```python
from build123d import *

# Parameters (mm, degrees)
F0_W     = 70
F0_H     = 100
F1_DEPTH = 10
F3_DEPTH = 70
F4_R     = 5
F6_D     = 11
F9_DEPTH = 17.2


with BuildPart() as f1:
    # F0 (on Front) → F1 (new body)
    with BuildSketch(Plane.XZ):
        with Locations((-0.1439042389, 3.7611486804)):
            Rectangle(F0_W, F0_H)
    extrude(amount=F1_DEPTH)

    # F2 (on face) → F3 (join)
    with BuildSketch(Plane.YZ.offset(34.8560957611)):
        with BuildLine():
            Line((-10, -46.2388513196), (-10, 53.7611486804))
            ThreePointArc((-10, 53.7611486804), (-21.8296936781, 3.7611486804), (-10, -46.2388513196))
        make_face()
    extrude(amount=-F3_DEPTH)

    # F4
    f4_edges = [f1.edges().sort_by_distance(p)[0] for p in [
        (34.856096, -5, 53.761149),
        (-35.143904, -5, 53.761149),
        (34.856096, -5, -46.238851),
        (-35.143904, -5, -46.238851),
    ]]
    fillet(f4_edges, radius=F4_R)

    # F6 (through all)
    with Locations(Plane(origin=(0, 0, 0), x_dir=(1, 0, 0), z_dir=(0, 1, 0))):
        with Locations((0, -33.7616663978), (0, -21.2616663978), (0, 13.7393690371), (0, 26.2393690371)):
            Hole(F6_D / 2)

    # F8 (on offset) → F9 (cut)
    with BuildSketch(Plane.XZ.offset(23.6)):
        with BuildLine():
            ThreePointArc((5.1695684419, 28.491923844), (-0.1945076363, 41.3073727185), (-4.8824502155, 28.2294433564))
            ThreePointArc((-4.8824502155, 28.2294433564), (-4.1963299736, 27.5433231145), (-4.8824502155, 26.8572028726))
            ThreePointArc((-4.8824502155, 26.8572028726), (-0.17230498, 13.7974067448), (5.2084099632, 26.5955179234))
            ThreePointArc((5.2084099632, 26.5955179234), (4.2211666178, 27.5238982808), (5.1695684419, 28.491923844))
        make_face()
        with BuildLine():
            ThreePointArc((5.1695684419, -19.5465231666), (-0.1945076363, -6.7310742921), (-4.8824502155, -19.8090036542))
            ThreePointArc((-4.8824502155, -19.8090036542), (-4.1963299736, -20.4951238961), (-4.8824502155, -21.181244138))
            ThreePointArc((-4.8824502155, -21.181244138), (-0.17230498, -34.2410402658), (5.2084099632, -21.4429290872))
            ThreePointArc((5.2084099632, -21.4429290872), (4.2211666178, -20.5145487298), (5.1695684419, -19.5465231666))
        make_face()
    extrude(amount=-F9_DEPTH, mode=Mode.SUBTRACT)


solid = f1.part
```
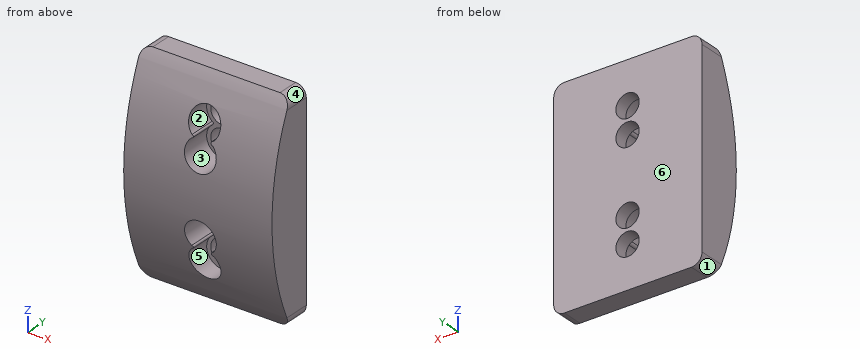
Here's how the part is built. I have some questions about the finished solid (model axes, mm). Face numbers are marked on the shaded views. A direction names the side the tool comes from. Give positions to 0.01 mm unless a question says otherwise; leave off trailing zeros. Loops run counter-clockwise (first coordinate to the right, second up) from the corner with the lowest first, then second, coordinate; pieces in that order, holes last. Notation, with made-up numbers: (74, 25.5) -> (107, 25.5) arc R31 ccw to (107, 49.5) -> close; hole circle Ø4 at (-8, 84.5). An arc over 180 degrees is marked (long way). Use one line per item in the form item = value. Start each with the question number.
1) Which directions (+Z, -Z, +X, -X, +Y, -Y) give clear straight access to the entire face, cutting with the end or side of a thin tool? Please do the marked faces 5 and 6.
2) For P1, Ø13.5, axis at x = 0.02, z = 21.25, coming from the -Y side; P2, Ø7.5, axis at x = -3.5, z = -18.5, coming from the -Y side; P3, Ø7.5, axis at x = -2, z = 29, coming from the -Y side; P4, Ø9, axis at x = 0, z = 21.26, coming from the -Y side, each with a flat end and sliding along its axis, tell me the tip position at first contact or that it passes through.
3) Imagine slicing it at B-B (x = 0). Please give me the cut outline in (y, z).
4) Please list where these lines run through material, in increasing order: line 1 along Z through (x, y) = (0, -4.5); line 2 along X through (y, z) = (-11, 34); line 3 along Z through (x, y) = (-0.5, -13).
5) Imagine slicing it at D-D (x = 11.5). Please give me the cut outline in (y, z), then the cut area to 3 significant figures.
6) Imagine slicing it at C-C (y = -4.5). Please give me the cut outline in (x, z), then the cut area to 3 significant figures.
7) Imagine slicing it at A-A (z = -11.5). Please give me the cut outline in (x, y), then the cut area to 3 significant figures.
8) Thinking about a two-plate mould opening in X: for the marked faces 1, 2, 3 and 4, which applies, +X half, -X half, draft (parallel to the pull), parting line (faces both ways), or undercut?
Check values:
q1.face_5 = -Y
q1.face_6 = +Z, -Z, +X, -X, +Y
q2.P1 = -6.4
q2.P2 = -19.89
q2.P3 = -19.44
q2.P4 = through
q3.outline = (-21.38, 13.79) arc R111.58 ccw to (-21.34, -6.73) -> (-6.4, -6.73) -> (-6.4, -8.24) -> (0, -8.24) -> (0, 15.76) -> (-6.4, 15.76) -> (-6.4, 13.79) -> close; (-15.32, 41.31) -> (-6.4, 41.31) -> (-6.4, 39.26) -> (0, 39.26) -> (0, 53.76) -> (-10, 53.76) arc R111.58 ccw to start; (-15.16, -34.24) arc R111.58 ccw to (-10, -46.24) -> (0, -46.24) -> (0, -31.74) -> (-6.4, -31.74) -> (-6.4, -34.24) -> close; (-6.4, -20.74) -> (0, -20.74) -> (0, -19.24) -> (-6.4, -19.24) -> close; (-6.4, 26.76) -> (0, 26.76) -> (0, 28.26) -> (-6.4, 28.26) -> close
q4.line_1 = -46.24 to -31.74, -20.74 to -19.24, -8.24 to 15.76, 26.76 to 28.26, 39.26 to 53.76
q4.line_2 = -35.14 to -7.45, 7.45 to 34.86
q4.line_3 = -39.74 to -34.23, -6.75 to 13.81, 41.29 to 47.26
q5.outline = (-10, -46.24) -> (0, -46.24) -> (0, 53.76) -> (-10, 53.76) arc R111.58 ccw to start
q5.area = 1,800 mm^2
q6.outline = (-35.14, -41.24) arc R5 ccw to (-30.14, -46.24) -> (29.86, -46.24) arc R5 ccw to (34.86, -41.24) -> (34.86, 48.76) arc R5 ccw to (29.86, 53.76) -> (-30.14, 53.76) arc R5 ccw to (-35.14, 48.76) -> close; hole circle Ø11 at (0, -26.24); hole circle Ø11 at (0, -13.74); hole circle Ø11 at (0, 21.26); hole circle Ø11 at (0, 33.76)
q6.area = 6,600 mm^2
q7.outline = (-35.14, -20.78) -> (-6.95, -20.78) -> (-6.95, -6.4) -> (-5.02, -6.4) -> (-5.02, 0) -> (-35.14, 0) -> close; (5.02, -6.4) -> (6.95, -6.4) -> (6.95, -20.78) -> (34.86, -20.78) -> (34.86, 0) -> (5.02, 0) -> close
q7.area = 1,190 mm^2
q8.face_1 = -X half
q8.face_2 = undercut
q8.face_3 = undercut
q8.face_4 = +X half
